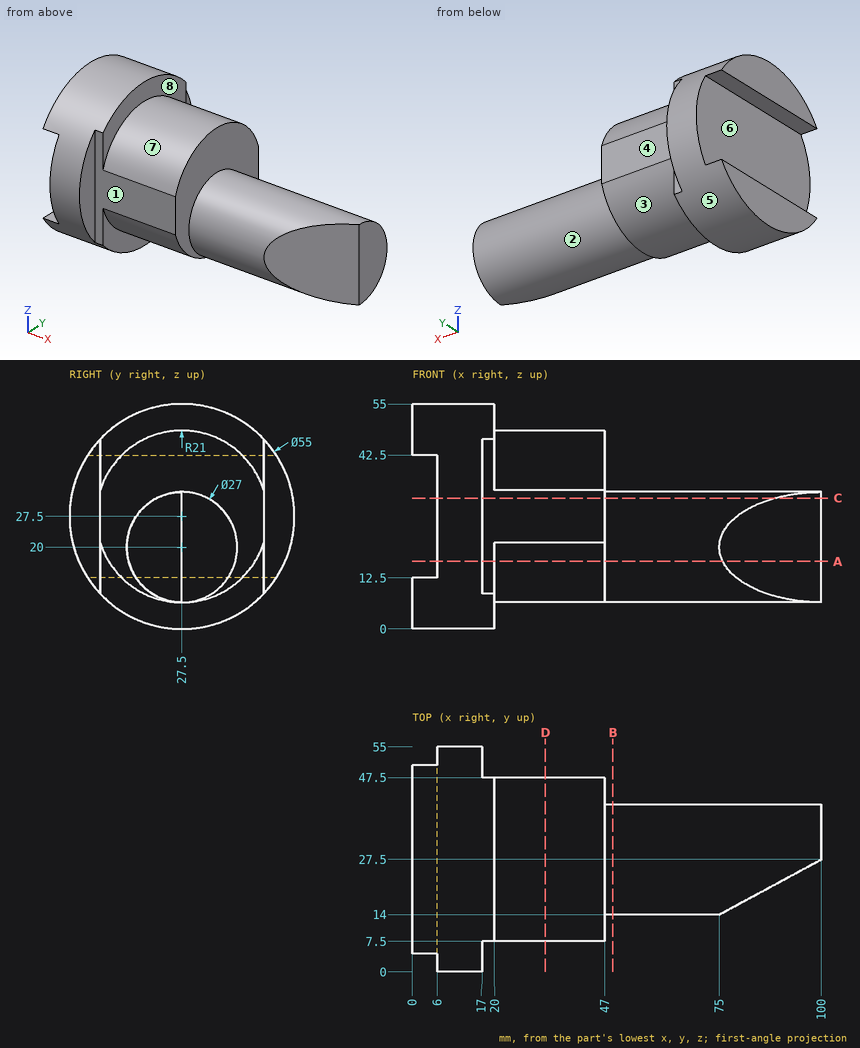
Study the drawing (mm; zero at the part's minimum x, y, z) and answer. A direction names the side the tool comes from. Give positions to 0.01 mm unless a question says otherwise; leave off trailing zeros. Loops run counter-clockwise (first coordinate to the right, second up) from the corner with the lowest first, then second, coordinate; pieces in that order, holes last. Notation, with made-up numbers: (-4, -27) - (46, -27) arc R22 ccw to (46, -18) - close; hole circle Ø10 at (-2.5, 65.5). An arc over 180 degrees is marked (long way). Return JSON: item names as keys, results as strings. Group by question number.
1. Which of the six approach directions +Z, -Z, +X, -X, +Y, -Y give full straight-line access (tool end or side, diameter ignored) to the marked faces 1, 2, 3 and 4?
2. Given pin 1 Ø5 at (x, y) = (2.5, 24) entering from +Z; pin 2 Ø9 at (x, z) = (25.5, 32.5) entering from -Y; pin 3 Ø4 at (y, z) = (2.5, 23) entering from +X; pin 4 Ø10 at (x, z) = (56.5, 39) entering from -Y, each flat-ended and moving along its own axis, determine where each tip first touches the part or whether it passes through.
3. Find section B-B (x = 49). Write down the section's boundary in (y, z).
4. Straight lines are drawn through the part: line 1 (X direction, y = 46, z = 33); line 2 (X direction, y = 9, z = 38.5); line 3 (Y direction, x = 33, z = 27.5). For each, find the intervals that lie inside material, in ascending order. Write a range as [from, to].
5. Determine the mould class of the marked faces 5, 6, 7 and 8 for opening direction Z: pulls with the +Z half, pulls with the -Z half, needs draft (parallel to the pull), parting line crosses it, or undercut.
6. Find section D-D (x = 32.5). Write down the section's boundary in (y, z).
7. Find section C-C (z = 32). Write down the section's boundary in (x, y), then the cut area to 3 significant figures.
8. Find section A-A (z = 16.5). Write down the section's boundary in (x, y), then the cut area to 3 significant figures.
Verdict:
{
 "1": {"face 1": "+Z, -Z, +X, -Y", "face 2": "+X", "face 3": "-Z, +X", "face 4": "+Z, -Z, +X, +Y"},
 "2": {"pin 1": "stops at z = 54.98", "pin 2": "stops at y = 7.5", "pin 3": "stops at x = 17", "pin 4": "passes through"},
 "3": {"outline": "circle Ø27 at (27.5, 20)"},
 "4": {"line 1": "x = [6, 47]", "line 2": "x = [6, 20]", "line 3": "y = [7.5, 47.5]"},
 "5": {"face 5": "parting line crosses it", "face 6": "undercut", "face 7": "pulls with the +Z half", "face 8": "needs draft"},
 "6": {"outline": "(7.5, 21.1) arc R21 ccw to (47.5, 21.1) - (47.5, 33.9) arc R21 ccw to (7.5, 33.9) - close"},
 "7": {"outline": "(6, 0.37) - (17, 0.37) - (17, 7.5) - (47, 7.5) - (47, 21.32) - (88.55, 21.32) - (100, 27.5) - (100, 33.68) - (47, 33.68) - (47, 47.5) - (17, 47.5) - (17, 54.63) - (6, 54.63) - close", "area": "2,420 mm^2"},
 "8": {"outline": "(6, 2.3) - (17, 2.3) - (17, 7.5) - (20, 7.5) - (20, 9.61) - (47, 9.61) - (47, 14.46) - (75.85, 14.46) - (100, 27.5) - (100, 40.54) - (47, 40.54) - (47, 45.39) - (20, 45.39) - (20, 47.5) - (17, 47.5) - (17, 52.7) - (6, 52.7) - close", "area": "2,870 mm^2"}
}
